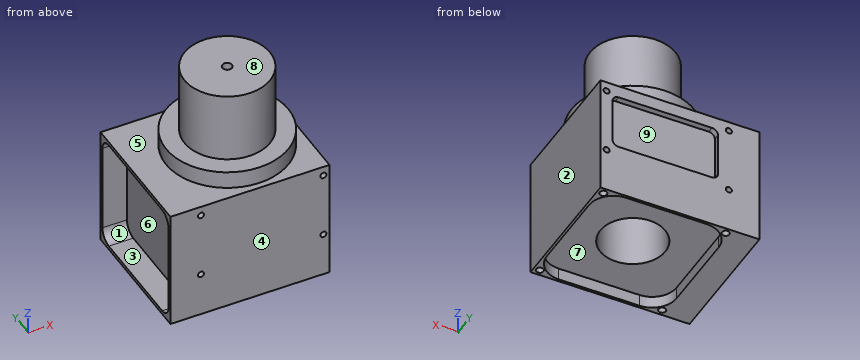
from build123d import *

# Parameters (mm, degrees)
SKETCH1_W           = 130
SKETCH1_H           = 100
SKETCH1_R           = 2.5
BOSS_EXTRUDE1_DEPTH = 110
CUT_EXTRUDE1_DEPTH  = 5
SKETCH3_R           = 26.593196083
CUT_EXTRUDE2_DEPTH  = 90
SKETCH4_R           = 3
CUT_EXTRUDE3_DEPTH  = 10
CUT_EXTRUDE4_DEPTH  = 20
SKETCH8_R           = 10
CUT_EXTRUDE5_DEPTH  = 10
SKETCH9_R           = 50
SKETCH9_R_2         = 14.996239462
BOSS_EXTRUDE3_DEPTH = 14.5
SKETCH10_R          = 35
SKETCH10_R_2        = 4
BOSS_EXTRUDE4_DEPTH = 58.5


with BuildPart() as part:
    # Sketch1 → Boss-Extrude1 (new body)
    with BuildSketch(Plane(origin=(0, 0, 0), x_dir=(1, 0, 0), z_dir=(0, 1, 0))):
        with Locations((65, -50)):
            Rectangle(SKETCH1_W, SKETCH1_H)
        with Locations(Location((25, -37, 0), (0, 0, 270))):  # turned: the seam where the file's is
            Circle(SKETCH1_R, mode=Mode.SUBTRACT)
        with Locations(Location((25, -92, 0), (0, 0, 270))):  # turned: the seam where the file's is
            Circle(SKETCH1_R, mode=Mode.SUBTRACT)
        with Locations(Location((125, -37, 0), (0, 0, 270))):  # turned: the seam where the file's is
            Circle(SKETCH1_R, mode=Mode.SUBTRACT)
        with Locations(Location((125, -92, 0), (0, 0, 270))):  # turned: the seam where the file's is
            Circle(SKETCH1_R, mode=Mode.SUBTRACT)
    extrude(amount=BOSS_EXTRUDE1_DEPTH)

    # Sketch2 → Cut-Extrude1 (cut)
    with BuildSketch(Plane(origin=(0, 110, 0), x_dir=(1, 0, 0), z_dir=(0, 1, 0))):
        with BuildLine():
            Line((38.9, -43.4), (115.1, -43.4))
            ThreePointArc((115.1, -43.4), (118.635533906, -44.864466094), (120.1, -48.4))
            Line((120.1, -48.4), (120.1, -84.6))
            ThreePointArc((120.1, -84.6), (118.635533906, -88.135533906), (115.1, -89.6))
            Line((115.1, -89.6), (38.9, -89.6))
            ThreePointArc((38.9, -89.6), (35.364466094, -88.135533906), (33.9, -84.6))
            Line((33.9, -84.6), (33.9, -48.4))
            ThreePointArc((33.9, -48.4), (35.364466094, -44.864466094), (38.9, -43.4))
        make_face()
    extrude(amount=-CUT_EXTRUDE1_DEPTH, mode=Mode.SUBTRACT)

    # Sketch3 → Cut-Extrude2 (cut)
    with BuildSketch(Plane(origin=(0, 0, 0), x_dir=(-1, 0, 0), z_dir=(0, 0, -1))):
        with Locations((-75, 55)):
            Circle(SKETCH3_R)
    extrude(amount=-CUT_EXTRUDE2_DEPTH, mode=Mode.SUBTRACT)

    # Sketch4 → Cut-Extrude3 (cut)
    with BuildSketch(Plane(origin=(0, 0, 0), x_dir=(-1, 0, 0), z_dir=(0, 0, -1))):
        with Locations((-125, 105)):
            Circle(SKETCH4_R)
        with Locations((-25, 105)):
            Circle(SKETCH4_R)
        with Locations((-125, 5)):
            Circle(SKETCH4_R)
        with Locations((-25, 5)):
            Circle(SKETCH4_R)
        with BuildLine():
            Line((-108, 108), (-42, 108))
            ThreePointArc((-42, 108), (-27.857864376, 102.142135624), (-22, 88))
            Line((-22, 88), (-22, 22))
            ThreePointArc((-22, 22), (-27.857864376, 7.857864376), (-42, 2))
            Line((-42, 2), (-108, 2))
            ThreePointArc((-108, 2), (-122.142135624, 7.857864376), (-128, 22))
            Line((-128, 22), (-128, 88))
            ThreePointArc((-128, 88), (-122.142135624, 102.142135624), (-108, 108))
        make_face()
    extrude(amount=-CUT_EXTRUDE3_DEPTH, mode=Mode.SUBTRACT)

    # Sketch6 → Cut-Extrude4 (cut)
    with BuildSketch(Plane.ZY):
        with BuildLine():
            Line((3, 13), (3, 97))
            ThreePointArc((3, 97), (5.928932188, 104.071067812), (13, 107))
            Line((13, 107), (87, 107))
            ThreePointArc((87, 107), (94.071067812, 104.071067812), (97, 97))
            Line((97, 97), (97, 13))
            ThreePointArc((97, 13), (94.071067812, 5.928932188), (87, 3))
            Line((87, 3), (13, 3))
            ThreePointArc((13, 3), (5.928932188, 5.928932188), (3, 13))
        make_face()
    extrude(amount=-CUT_EXTRUDE4_DEPTH, mode=Mode.SUBTRACT)

    # Sketch8 → Cut-Extrude5 (cut)
    with BuildSketch(Plane.XY.offset(100)):
        with Locations((75, 55)):
            Circle(SKETCH8_R)
    extrude(amount=-CUT_EXTRUDE5_DEPTH, mode=Mode.SUBTRACT)

    # Sketch9 → Boss-Extrude3 (add)
    with BuildSketch(Plane.XY.offset(100)):
        with Locations(Location((75, 55, 0), (0, 0, 180))):  # turned: the seam where the file's is
            Circle(SKETCH9_R)
        with Locations((75, 55)):
            Circle(SKETCH9_R_2, mode=Mode.SUBTRACT)
    extrude(amount=BOSS_EXTRUDE3_DEPTH)

    # Sketch10 → Boss-Extrude4 (add)
    with BuildSketch(Plane.XY.offset(114.5)):
        with Locations((75, 55)):
            Circle(SKETCH10_R)
        with Locations((75, 55)):
            Circle(SKETCH10_R_2, mode=Mode.SUBTRACT)
    extrude(amount=BOSS_EXTRUDE4_DEPTH)


solid = part.part
Design review of the part built by this model. Coordinates are the model's own, in mm. Face numbers are marked on the shaded views. A direction names the side the tool comes from. Coordinates: 2 decimals unless noted, no trailing zeros. Loops run counter-clockwise (first coordinate to the right, second up) from the corner with the lowest first, then second, coordinate; pieces in that order, holes last. Notation, with made-up numbers: (8.5, -8) -> (39.5, -8) arc R37 ccw to (39.5, 28) -> close; hole circle Ø5 at (20.25, 87). An arc over 180 degrees is marked (long way). Use a Markdown table: item, result. Add a question column.
Item 1: Machinability: for the marked faces 5, 6, 7, 8 and 9, which of the approach directions +Z, -Z, +X, -X, +Y, -Y give a long, thin tool a straight path to every point of the face, cutting with its end or side? Answer none if there is none.
Item 2: We need section A-A, the plane z = 37. Write out the cut boundary in (x, y).
Item 3: We need section B-B, the plane x = 15.5. Write out the cut boundary in (y, z), and give its area (3 significant figures).
Item 4: We need section C-C, the plane y = 55. Count the separate pieces of the cut face and the enclosed holes in it, and give its area (3 significant figures).
Item 5: Wall thickness on L1, parallel to Z at x = 10.5, y = 70.5; L2, parallel to Y at x = 75, z = 27; L3, parallel to Z at x = 26, y = 84: over which ranges is each line inside the solid? List them lowest first. Write a range as from..to.
Item 6: Clearance check with flat-ended pins moving along their axes: P1, Ø5, axis at x = 125, y = 5, coming from the +Z side; P2, Ø1.5, axis at x = 102, y = 17, coming from the +Z side; P3, Ø23, axis at x = 60.5, z = 62.5, coming from the +Y side. State where each tip first meets the part, or that it passes through.
Item 7: The part is to be moulded in two halves that separate along Y. For the marked faces 1, 2, 3 and 4, say which applies: +Y half, -Y half, draft (parallel to the pull), parting line (faces both ways), or undercut.
Item 8: We need section D-D, the plane y = 24.5. Write out the cut boundary in (x, z).
Numbers:
| question | item | result |
|---|---|---|
| 1 | face 5 | +Z |
| 1 | face 6 | -X |
| 1 | face 7 | -Z |
| 1 | face 8 | +Z, +X, -X, +Y, -Y |
| 1 | face 9 | +Y |
| 2 | outline | (0, 0) -> (22.5, 0) -> (22.5, 110) -> (0, 110) -> (0, 107) -> (20, 107) -> (20, 3) -> (0, 3) -> close; (27.5, 0) -> (122.5, 0) -> (122.5, 110) -> (27.5, 110) -> close; (127.5, 0) -> (130, 0) -> (130, 110) -> (127.5, 110) -> close; hole circle Ø53.19 at (75, 55) |
| 3 | outline | (0, 0) -> (110, 0) -> (110, 100) -> (0, 100) -> close; hole (3, 13) arc R10 ccw to (13, 3) -> (97, 3) arc R10 ccw to (107, 13) -> (107, 87) arc R10 ccw to (97, 97) -> (13, 97) arc R10 ccw to (3, 87) -> close |
| 3 | area | 1,310 mm^2 |
| 4 | separate pieces | 2 |
| 4 | enclosed holes | 4 |
| 4 | area | 10,200 mm^2 |
| 5 | L1 | z = 0..3, 97..100 |
| 5 | L2 | y = 0..28.41, 81.59..110 |
| 5 | L3 | z = 10..34.71, 39.29..89.71, 94.29..100 |
| 6 | P1 | stops at z = 100 |
| 6 | P2 | stops at z = 114.5 |
| 6 | P3 | stops at y = 105 |
| 7 | face 1 | undercut |
| 7 | face 2 | draft |
| 7 | face 3 | undercut |
| 7 | face 4 | -Y half |
| 8 | outline | (0, 0) -> (22, 0) -> (22, 10) -> (128, 10) -> (128, 0) -> (130, 0) -> (130, 100) -> (114.62, 100) -> (114.62, 114.5) -> (92.17, 114.5) -> (92.17, 173) -> (57.83, 173) -> (57.83, 114.5) -> (35.38, 114.5) -> (35.38, 100) -> (0, 100) -> (0, 97) -> (20, 97) -> (20, 3) -> (0, 3) -> close; hole circle Ø5 at (25, 37); hole circle Ø5 at (25, 92); hole circle Ø5 at (125, 37); hole circle Ø5 at (125, 92) |
